from build123d import *

# Parameters (mm, degrees)
F0_R          = 6
F1_DEPTH      = 10
F0_R_2        = 30
F2_DEPTH      = 4
F3_R          = 1.5
F4_DEPTH      = 25.3
F4_DEPTH_BACK = 25
F6_DEPTH      = 9.4
F11_DEPTH     = 25


with BuildPart() as f1:
    # F0 (on Front) → F1 (new body)
    with BuildSketch(Plane.XZ):
        Circle(F0_R)
    extrude(amount=F1_DEPTH)

    # F0 (on Front) → F2 (join)
    with BuildSketch(Plane.XZ):
        Circle(F0_R_2)
        Circle(F0_R, mode=Mode.SUBTRACT)
    extrude(amount=F2_DEPTH)

    # F3 (on Right) → F4 (cut, two sides)
    with BuildSketch(Plane.YZ) as f4_sk:
        with Locations((-6.6611841321, 0)):
            Circle(F3_R)
    extrude(amount=-F4_DEPTH, mode=Mode.SUBTRACT)
    extrude(f4_sk.sketch, amount=F4_DEPTH_BACK, mode=Mode.SUBTRACT)

    # F5 (on face) → F6 (cut)
    with BuildSketch(Plane.XZ.offset(10)):
        with BuildLine():
            ThreePointArc((-1.5, -2.3), (0, -2.7459060435), (1.5, -2.3))
            Line((1.5, -2.3), (1.5, 2.3))
            ThreePointArc((1.5, 2.3), (0, 2.7540939565), (-1.5, 2.3))
            Line((-1.5, 2.3), (-1.5, -2.3))
        make_face()
    extrude(amount=-F6_DEPTH, mode=Mode.SUBTRACT)

    # F7 (on Right) → F8 (revolve, cut)
    with BuildSketch(Plane.YZ):
        Polygon((-3.4562557703, -30), (-0.6278286455, -30), (-2.0420422079, -28.5857864376), align=None)
    revolve(axis=Axis((0, -4.137200769, 0), (0, 1, 0)), mode=Mode.SUBTRACT)

    # F10 (on face) → F11 (cut)
    with BuildSketch(Plane.XZ.offset(4)):
        with BuildLine():
            Line((0, -12.5489194834), (-14.2731177399, -22.9189465287))
            ThreePointArc((-14.2731177399, -22.9189465287), (0, -27), (14.2731177399, -22.9189465287))
            Line((14.2731177399, -22.9189465287), (0, -12.5489194834))
        make_face()
        with BuildLine():
            ThreePointArc((-26.207849387, 6.4921976638), (-25.5345752261, -8.7741363121), (-16.6820319121, -21.2299272558))
            Line((-16.6820319121, -21.2299272558), (-11.2141093823, -4.4013921035))
            Line((-11.2141093823, -4.4013921035), (-26.207849387, 6.4921976638))
        make_face()
        with BuildLine():
            ThreePointArc((-1.0174091694, 26.9808242754), (-16.0079494962, 21.7427126396), (-25.4614935227, 8.9840050977))
            Line((-25.4614935227, 8.9840050977), (-6.8649301898, 8.9840050977))
            Line((-6.8649301898, 8.9840050977), (-1.0174091694, 26.9808242754))
        make_face()
        with BuildLine():
            ThreePointArc((25.4614935227, 8.9840050977), (16.0079494962, 21.7427126396), (1.0174091694, 26.9808242754))
            Line((1.0174091694, 26.9808242754), (6.8649301898, 8.9840050977))
            Line((6.8649301898, 8.9840050977), (25.4614935227, 8.9840050977))
        make_face()
        with BuildLine():
            Line((11.2141093823, -4.4013921035), (16.6820319121, -21.2299272558))
            ThreePointArc((16.6820319121, -21.2299272558), (24.2838924148, -11.8022272977), (27, 0))
            ThreePointArc((27, 0), (26.8012306942, 3.270173279), (26.207849387, 6.4921976638))
            Line((26.207849387, 6.4921976638), (11.2141093823, -4.4013921035))
        make_face()
    extrude(amount=-F11_DEPTH, mode=Mode.SUBTRACT)


solid = f1.part
CAD build for the part. Positions are in the model's coordinates, mm. A direction names the side the tool comes from. Round coordinates to 2 decimals unless told otherwise and drop trailing zeros. Write each loop counter-clockwise with the first axis right and the second up, starting at its lowest first coordinate (ties: lowest second). Pieces come first, ordered by that corner, then holes. Notation, with made-up numbers: M 18.5,-15.75 L 26.5,-15.75 A12 cw 26.5,-4.75 Z; hole C 72.5,12 d2. An arc over 180 degrees is marked long. Use a Markdown table: item, result. Add a question column.
1. Slice it at A-A on y = -9. Give the cut face in (x, z).
2. Flat gauge pins, fed straight in: P1, Ø2.5, axis at x = 0, z = 0.5, coming from the -Y side; P2, Ø18, axis at x = -13, z = 10.5, coming from the -Y side; P3, Ø1.2, axis at x = 16, y = -2, coming from the +Z side. Where does each tip first touch, or does it go through?
3. Slice it at B-B on x = 3.5. Give the number of separate pieces and of enclosed holes in the cut face, then the cut area to 3 significant figures.
4. Pull direction X, two halves, no side cores. Call faces 4 (the face through (-0.4, -4, -6.2)), 5 (the face through (16.2, -2, 21.6)): released by +X, released by -X, zero draft, split by the parting line, or undercut.
5. Drill centre lines: probe 1 along Y at (x, z) = (3, 0); probe 2 along X at (y, z) = (-3.75, 13); probe 3 along X at (y, z) = (-1.75, -15). Where is each one in solid material? Low to high.
6. 3-axis set-ups, long thin cutter, end or side, ignore diameter. For faces 1 (the face through (3.72, -8.16, 0.07)), 2 (the face through (-18.61, -2.03, 0.97)), 3 (the face through (0.022, -5.366, 2.754)): which of +Z, -Z, +X, -X, +Y, -Y reach the whole face in a straight line?
Reply:
| question | item | result |
|---|---|---|
| 1 | outline | C 0,0 d12; hole M -1.5,-2.3 A2.75 ccw 1.5,-2.3 L 1.5,2.3 A2.7 ccw -1.5,2.3 Z |
| 2 | P1 | stops at y = -0.6 |
| 2 | P2 | stops at y = -4 |
| 2 | P3 | stops at z = 24.56 |
| 3 | separate pieces | 3 |
| 3 | enclosed holes | 1 |
| 3 | area | 209 mm^2 |
| 4 | face 4 | zero draft |
| 4 | face 5 | undercut |
| 5 | probe 1 | y = -10 to -8.16, -5.16 to 0 |
| 5 | probe 2 | x = -27.04 to -23.66, -5.56 to 5.56, 23.66 to 27.04 |
| 5 | probe 3 | x = -24.68 to -22.45, -14.66 to -3.37, 3.37 to 14.66, 22.45 to 24.68 |
| 6 | face 1 | +X, -X |
| 6 | face 2 | +Y, -Y |
| 6 | face 3 | -Y |
